The listing builds one solid part. Answer for the finished solid, in the listing's coordinates (mm). A direction names the side the tool comes from. Coordinates: 2 decimals unless noted, no trailing zeros. Order: outer loops, then holes, each group sorted by start corner. A loop starts at its lowest first (then second) coordinate and runs counter-clockwise, first axis right, second up. Notation, with made-up numbers: (-18, -8.5) -> (-11, -8.5) arc R23 ccw to (-11, 20.5) -> close; hole circle Ø6 at (13.25, -24). An arc over 180 degrees is marked (long way). Write item = value, one per line.
from build123d import *

# Parameters (mm, degrees)
SKETCH1_R           = 1.27
BOSS_EXTRUDE2_DEPTH = 1.5875
SKETCH6_W           = 2.032
SKETCH6_H           = 7.366
CUT_EXTRUDE4_DEPTH  = 2.54
SKETCH7_R           = 1
CUT_EXTRUDE5_DEPTH  = 2.54


with BuildPart() as part:
    # Sketch1 → Boss-Extrude2 (new body)
    with BuildSketch(Plane(origin=(0, 0, 0), x_dir=(1, 0, 0), z_dir=(0, 1, 0))):
        with BuildLine():
            Line((-41.794385987, 35.56), (0, 11.43))
            Line((0, 11.43), (0, 0))
            Line((0, 0), (17.78, 0))
            Line((17.78, 0), (17.78, -67.587878735))
            Line((17.78, -67.587878735), (33.02, -67.587878735))
            Line((33.02, -67.587878735), (33.02, 0))
            Line((33.02, 0), (50.8, 0))
            Line((50.8, 0), (50.8, 11.43))
            Line((50.8, 11.43), (92.594385987, 35.56))
            Line((92.594385987, 35.56), (84.974385987, 48.758227154))
            Line((84.974385987, 48.758227154), (43.18, 24.628227154))
            Line((43.18, 24.628227154), (30.9, 24.628227154))
            Line((30.9, 24.628227154), (30.9, 18.264121265))
            ThreePointArc((30.9, 18.264121265), (25.4, 12.764121265), (19.9, 18.264121265))
            Line((19.9, 18.264121265), (19.9, 24.628227154))
            Line((19.9, 24.628227154), (7.62, 24.628227154))
            Line((7.62, 24.628227154), (-34.174385987, 48.758227154))
            Line((-34.174385987, 48.758227154), (-41.794385987, 35.56))
        make_face()
        with Locations(Location((43.690443212, 16.124113577, 0), (0, 0, 270))):
            Circle(SKETCH1_R, mode=Mode.SUBTRACT)
        with Locations(Location((36.398522628, 11.914121265, 0), (0, 0, 270))):
            Circle(SKETCH1_R, mode=Mode.SUBTRACT)
        with Locations(Location((14.401477372, 11.914121265, 0), (0, 0, 270))):
            Circle(SKETCH1_R, mode=Mode.SUBTRACT)
        with Locations(Location((7.109556788, 16.124113577, 0), (0, 0, 270))):
            Circle(SKETCH1_R, mode=Mode.SUBTRACT)
        with Locations(Location((10.409113577, 14.219113577, 0), (0, 0, 270))):
            Circle(SKETCH1_R, mode=Mode.SUBTRACT)
        with Locations(Location((40.390886423, 14.219113577, 0), (0, 0, 270))):
            Circle(SKETCH1_R, mode=Mode.SUBTRACT)
        with Locations(Location((25.4, -7.135878735, 0), (0, 0, 270))):
            Circle(SKETCH1_R, mode=Mode.SUBTRACT)
        with Locations(Location((25.4, -15.517878735, 0), (0, 0, 270))):
            Circle(SKETCH1_R, mode=Mode.SUBTRACT)
        with Locations(Location((25.4, -11.707878735, 0), (0, 0, 270))):
            Circle(SKETCH1_R, mode=Mode.SUBTRACT)
    extrude(amount=BOSS_EXTRUDE2_DEPTH)

    # Sketch6 → Cut-Extrude4 (cut)
    with BuildSketch(Plane(origin=(0, 0, 0), x_dir=(-1, 0, 0), z_dir=(0, -1, 0))):
        with Locations((-18.796, -7.008878735)):
            Rectangle(SKETCH6_W, SKETCH6_H)
    extrude(amount=-CUT_EXTRUDE4_DEPTH, mode=Mode.SUBTRACT)

    # Sketch7 → Cut-Extrude5 (cut)
    with BuildSketch(Plane(origin=(0, 0, 0), x_dir=(-1, 0, 0), z_dir=(0, -1, 0))):
        with Locations(Location((-25.4, -59.967878735, 0), (0, 0, 90))):
            Circle(SKETCH7_R)
        with Locations(Location((-25.4, -47.267878735, 0), (0, 0, 90))):
            Circle(SKETCH7_R)
        with Locations(Location((-71.186749782, 31.999113577, 0), (0, 0, 90))):
            Circle(SKETCH7_R)
        with Locations(Location((-82.18527241, 38.349113577, 0), (0, 0, 90))):
            Circle(SKETCH7_R)
        with Locations(Location((31.38527241, 38.349113577, 0), (0, 0, 90))):
            Circle(SKETCH7_R)
        with Locations(Location((20.386749782, 31.999113577, 0), (0, 0, 90))):
            Circle(SKETCH7_R)
    extrude(amount=-CUT_EXTRUDE5_DEPTH, mode=Mode.SUBTRACT)


solid = part.part
Q1. A tool of negligible diameter and unlimited length cuts with its end or side. For faces 4 (the face through (-12.98, 0.78, -36.52)), 5 (the face through (-21.19, 0.783, -23.664)), from which of +Z, -Z, +X, -X, +Y, -Y can it reach the whole face along a straight path? Write none if from no direction.
The answers:
face_4 = -Z, +Y, -Y
face_5 = +Z, -X, +Y, -Y
Q2. Section B-B, the plane z = 44 is taken. Give the vertices of the cut face in (x, y), plus the area to 3 significant figures.
The answers:
outline = (17.78, 0) -> (33.02, 0) -> (33.02, 1.59) -> (17.78, 1.59) -> close
area = 24.2 mm2
Q3. Section C-C, the plane y = 1.05 is taken. Give the number of separate pieces and of enclosed holes in the cut face, plus the area to 3 significant figures.
The answers:
separate_pieces = 1
enclosed_holes = 15
area = 3,450 mm2
Q4. Each of these flat-tipped pins is pushed along its axis until it touches: pin 1 Ø0.8 at (x, y) = (14.5, 1) entering from -Z; pin 2 Ø0.5 at (x, y) = (10, 1) entering from +Z; pin 3 Ø1.8 at (x, z) = (82.19, -38.35) entering from +Y; pin 4 Ø3.5 at (x, z) = (40.39, -14.22) entering from +Y. Where does it stop, or does it pass through?
The answers:
pin_1 = -24.63
pin_2 = 0
pin_3 = through
pin_4 = 1.59
Q5. Section A-A, the plane z = -27 is taken. Give the vertices of the cut face in (x, y).
The answers:
outline = (-26.97, 0) -> (3.51, 0) -> (3.51, 1.59) -> (-26.97, 1.59) -> close; (47.29, 0) -> (77.77, 0) -> (77.77, 1.59) -> (47.29, 1.59) -> close
Q6. Find the intervals of material crossed by line 1 along X through (y, z) = (0.45, -12.5); line 2 along X through (y, z) = (0.95, -7); line 3 along X through (y, z) = (0.2, 43), in increasing order.
The answers:
line_1 = -1.85 to 13.27, 15.53 to 35.27, 37.53 to 52.65
line_2 = 0 to 50.8
line_3 = 17.78 to 33.02
Q7. Section D-D, the plane x = 75.5 is taken. Give the vertices of the cut face in (y, z), plus the area to 3 significant figures.
The answers:
outline = (0, -43.29) -> (1.59, -43.29) -> (1.59, -25.69) -> (0, -25.69) -> close
area = 27.9 mm2
Q8. The mould has two halves that part along X. Classify faces 1 (the face through (64.37, 0.78, -36.86)), 2 (the face through (-37.93, 0.78, -42.25)), 3 (the face through (71.405, 0.783, -23.326)): released by +X, released by -X, zero draft, split by the parting line, or undercut.
The answers:
face_1 = undercut
face_2 = released by -X
face_3 = released by +X
